Geometry: final body of the model. Coordinates: model frame, mm. A direction names the side the tool comes from. Give positions to 0.01 mm unless a question says otherwise; leave off trailing zeros. Write each loop counter-clockwise with the first axis right and the second up, starting at its lowest first coordinate (ties: lowest second). Pieces come first, ordered by that corner, then holes. Notation, with made-up numbers: (86.5, 53) - (112.5, 53) arc R14 cw to (112.5, 79) - close; hole circle Ø1 at (46.25, 6.5). An arc over 180 degrees is marked (long way). One line per question, with ' | ' between items. Start each with the question number.
```python
from build123d import *

# Parameters (mm, degrees)
SKETCH_R              = 35
PAD_DEPTH             = 30
SKETCH001_R           = 12
POCKET_DEPTH          = 30.001
SKETCH002_R           = 26
POCKET001_DEPTH       = 5
SKETCH003_R           = 3.25
POCKET002_DEPTH       = 15
POLARPATTERN_COUNT    = 16
SKETCH004_R           = 16
POCKET003_DEPTH       = 12
POCKET004_DEPTH       = 5
POLARPATTERN001_COUNT = 7


with BuildPart() as part:
    # Sketch → Pad (new body)
    with BuildSketch(Plane.XY):
        Circle(SKETCH_R)
    extrude(amount=PAD_DEPTH)

    # Sketch001 → Pocket (cut, through all)
    with BuildSketch(Plane(origin=(0, 0, 0), x_dir=(1, 0, 0), z_dir=(0, 0, -1))):
        Circle(SKETCH001_R)
    extrude(amount=-POCKET_DEPTH, mode=Mode.SUBTRACT)

    # Sketch002 → Pocket001 (cut)
    with BuildSketch(Plane(origin=(0, 0, 0), x_dir=(1, 0, 0), z_dir=(0, 0, -1))):
        Circle(SKETCH002_R)
    extrude(amount=-POCKET001_DEPTH, mode=Mode.SUBTRACT)

    # Sketch003 → Pocket002 (cut)
    with BuildSketch(Plane.XY.offset(30)):
        with Locations((0, 25)):
            Circle(SKETCH003_R)
    pocket002 = extrude(amount=-POCKET002_DEPTH, mode=Mode.SUBTRACT)

    # PolarPattern: Pocket002 ×16 about axis
    polarpattern_axis = Axis((0, 0, 30), (0, 0, 1))
    for i in range(1, POLARPATTERN_COUNT):
        add(pocket002.rotate(polarpattern_axis, i * 360 / POLARPATTERN_COUNT), mode=Mode.SUBTRACT)

    # Sketch004 → Pocket003 (cut)
    with BuildSketch(Plane.XY.offset(30)):
        Circle(SKETCH004_R)
    extrude(amount=-POCKET003_DEPTH, mode=Mode.SUBTRACT)

    # Sketch005 → Pocket004 (cut)
    with BuildSketch(Plane(origin=(0, 0, 0), x_dir=(1, 0, 0), z_dir=(0, 0, -1))):
        Polygon((19.471427, 37.015548), (21.112486, 34.504188), (-4.001108, 18.0936), (-5.642167, 20.604959), align=None)
    pocket004 = extrude(amount=-POCKET004_DEPTH, mode=Mode.SUBTRACT)

    # PolarPattern001: Pocket004 ×7 about axis
    polarpattern001_axis = Axis((0, 0, 0), (0, 0, -1))
    for i in range(1, POLARPATTERN001_COUNT):
        add(pocket004.rotate(polarpattern001_axis, i * 360 / POLARPATTERN001_COUNT), mode=Mode.SUBTRACT)


solid = part.part
```
1) Section D-D, the plane z = 20.75. Give the number of separate pieces and of enclosed holes in the cut face, plus the area to 3 significant figures.
2) Line query: L1, parallel to Y at x = 0, z = 23.75; L2, parallel to Y at x = -24, z = 23; L3, parallel to X at y = -7.5, z = 21. Output: solid intervals per line, ascending.
3) Section C-C, the plane x = 31.5. Output: boundary loops of the cut face in (y, z).
4) First-contact query: pin 1 Ø2 at (x, y) = (22.5, 10) entering from +Z; pin 2 Ø5 at (x, y) = (-23.5, -1.5) entering from +Z; pin 3 Ø16 at (x, y) = (6.5, -4) entering from +Z; pin 4 Ø12 at (y, z) = (-20, 11) entering from +X. Flat tips, straight axial feed; report the tip coordinate or a pass-through.
5) Pull-direction query (X, two-part tool) for faces 4 (the cylindrical face through (10.409, 26.236, 22.605)), 5 (the flat face through (17, 26, 0)); classes: +X half, -X half, draft (parallel to the pull), parting line (faces both ways), or undercut.
6) Reachability of faces 1 (the flat face through (-11, 29, 0)), 2 (the flat face through (26.796, 13.818, 2.465)), 3 (the flat face through (23, -10, 15)) from +Z, -Z, +X, -X, +Y, -Y: full face, straight path, thin tool, end or side. Return the list, or none.
7) Section A-A, the plane x = 0. Output: boundary loops of the cut face in (y, z), plus the area to 3 significant figures.
8) Section B-B, the plane z = 8.25. Output: boundary loops of the cut face in (x, y), plus the area to 3 significant figures.
Answer key:
1) separate pieces: 1 | enclosed holes: 17 | area: 2,510 mm^2
2) L1: -35 to -28.25, -21.75 to -16, 16 to 21.75, 28.25 to 35 | L2: -25.48 to -12.69, -6.45 to -3.09, 3.09 to 6.45, 12.69 to 25.48 | L3: -34.19 to -25.6, -20.59 to -14.13, 14.13 to 20.59, 25.6 to 34.19
3) outline: (-15.26, 0) - (-11.02, 0) - (-11.02, 5) - (-7.86, 5) - (-7.86, 0) - (15.26, 0) - (15.26, 30) - (-15.26, 30) - close
4) pin 1: z = 15 | pin 2: z = 30 | pin 3: z = 18 | pin 4: x = 32.08
5) face 4: undercut | face 5: draft
6) face 1: -Z, +X, -X, +Y, -Y | face 2: -Z | face 3: +Z
7) outline: (-35, 0) - (-26, 0) - (-26, 5) - (-12, 5) - (-12, 18) - (-16, 18) - (-16, 30) - (-21.75, 30) - (-21.75, 15) - (-28.25, 15) - (-28.25, 30) - (-35, 30) - close; (12, 5) - (26, 5) - (26, 0) - (33.54, 0) - (33.54, 5) - (35, 5) - (35, 30) - (28.25, 30) - (28.25, 15) - (21.75, 15) - (21.75, 30) - (16, 30) - (16, 18) - (12, 18) - close | area: 942 mm^2
8) outline: circle Ø70 at (0, 0); hole circle Ø24 at (0, 0) | area: 3,400 mm^2
